Design review of the part built by this model. Coordinates are the model's own, in mm. Coordinates: 2 decimals unless noted, no trailing zeros. Loops run counter-clockwise (first coordinate to the right, second up) from the corner with the lowest first, then second, coordinate; pieces in that order, holes last. Notation, with made-up numbers: (86, -3) -> (103, -3) arc R4 ccw to (103, 3) -> close; hole circle Ø6 at (45, 85.5). An arc over 180 degrees is marked (long way). Answer in a Markdown table with one row per item.
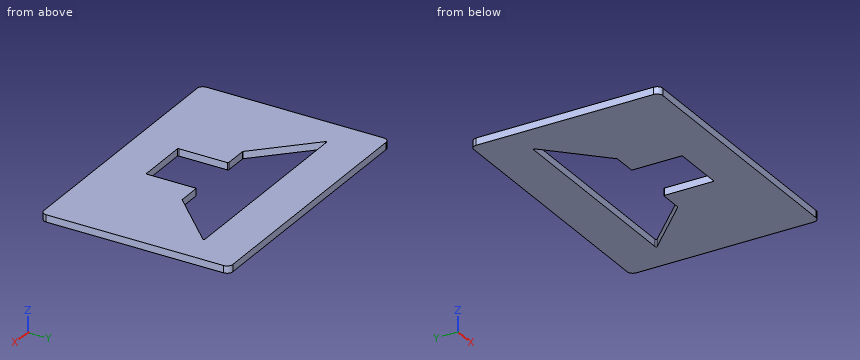
```python
from build123d import *

# Parameters (mm, degrees)
F1_DEPTH = 6.35
F3_DEPTH = 25.4
F5_DEPTH = 25.4


with BuildPart() as f1:
    # F0 (on Top) → F1 (new body)
    with BuildSketch(Plane.XY):
        with BuildLine():
            Line((113.9825, 84.1375), (-113.9825, 84.1375))
            ThreePointArc((-113.9825, 84.1375), (-117.574602, 82.649602), (-119.0625, 79.0575))
            Line((-119.0625, 79.0575), (-119.0625, -79.0575))
            ThreePointArc((-119.0625, -79.0575), (-117.574602, -82.649602), (-113.9825, -84.1375))
            Line((-113.9825, -84.1375), (113.9825, -84.1375))
            ThreePointArc((113.9825, -84.1375), (117.574602, -82.649602), (119.0625, -79.0575))
            Line((119.0625, -79.0575), (119.0625, 79.0575))
            ThreePointArc((119.0625, 79.0575), (117.574602, 82.649602), (113.9825, 84.1375))
        make_face()
    extrude(amount=F1_DEPTH)

    # F2 (on face) → F3 (cut)
    with BuildSketch(Plane.XY.offset(6.35)):
        Polygon((89.408, 43.8785), (0, 43.8785), (-89.408, 43.8785), (-44.45, -1.0795), (-22.479, -1.0795), (-22.479, -46.0375), (0, -46.0375), (22.479, -46.0375), (22.479, -1.0795), (44.45, -1.0795), align=None)
    extrude(amount=-F3_DEPTH, mode=Mode.SUBTRACT)

    # F4 (on face) → F5 (cut)
    with BuildSketch(Plane.XY.offset(6.35)):
        with BuildLine():
            ThreePointArc((-90.573099, 45.1485), (-91.300562, 44.662425), (-91.129875, 43.804324))
            Line((-91.129875, 43.804324), (-45.206675, -2.118876))
            ThreePointArc((-45.206675, -2.118876), (-44.951224, -2.289563), (-44.649899, -2.3495))
            Line((-44.649899, -2.3495), (-24.5364, -2.3495))
            ThreePointArc((-24.5364, -2.3495), (-23.979624, -2.580124), (-23.749, -3.1369))
            Line((-23.749, -3.1369), (-23.749, -46.5201))
            ThreePointArc((-23.749, -46.5201), (-23.518376, -47.076876), (-22.9616, -47.3075))
            Line((-22.9616, -47.3075), (22.9616, -47.3075))
            ThreePointArc((22.9616, -47.3075), (23.518376, -47.076876), (23.749, -46.5201))
            Line((23.749, -46.5201), (23.749, -3.1369))
            ThreePointArc((23.749, -3.1369), (23.979624, -2.580124), (24.5364, -2.3495))
            Line((24.5364, -2.3495), (44.649899, -2.3495))
            ThreePointArc((44.649899, -2.3495), (44.951224, -2.289563), (45.206675, -2.118876))
            Line((45.206675, -2.118876), (91.129875, 43.804324))
            ThreePointArc((91.129875, 43.804324), (91.300562, 44.662425), (90.573099, 45.1485))
            Line((90.573099, 45.1485), (-90.573099, 45.1485))
        make_face()
    extrude(amount=-F5_DEPTH, mode=Mode.SUBTRACT)


solid = f1.part
```
(1) To check wall thickness, follow probe 1 along Y at (x, z) = (-42, 3.5); probe 2 along Y at (x, z) = (19, 4.75); probe 3 along X at (y, z) = (20, 2.25). State the ranges of each line that lie inside material, in increasing order.
Evaluation:
| item | result |
|---|---|
| probe 1 | y = -84.14 to -2.35, 45.15 to 84.14 |
| probe 2 | y = -84.14 to -47.31, 45.15 to 84.14 |
| probe 3 | x = -119.06 to -67.33, 67.33 to 119.06 |
(2) Take a section at A-A on y = -32. Give the boundary of the cut face in (x, z), and give its area (3 significant figures).
Evaluation:
| item | result |
|---|---|
| outline | (-119.06, 0) -> (-23.75, 0) -> (-23.75, 6.35) -> (-119.06, 6.35) -> close; (23.75, 0) -> (119.06, 0) -> (119.06, 6.35) -> (23.75, 6.35) -> close |
| area | 1,210 mm² |
(3) Take a section at C-C on z = 2.5. Give the boundary of the cut face in (x, y), and give its area (3 significant figures).
Evaluation:
| item | result |
|---|---|
| outline | (-119.06, -79.06) arc R5.08 ccw to (-113.98, -84.14) -> (113.98, -84.14) arc R5.08 ccw to (119.06, -79.06) -> (119.06, 79.06) arc R5.08 ccw to (113.98, 84.14) -> (-113.98, 84.14) arc R5.08 ccw to (-119.06, 79.06) -> close; hole (-91.13, 43.8) -> (-45.21, -2.12) arc R0.79 ccw to (-44.65, -2.35) -> (-24.54, -2.35) arc R0.79 cw to (-23.75, -3.14) -> (-23.75, -46.52) arc R0.79 ccw to (-22.96, -47.31) -> (22.96, -47.31) arc R0.79 ccw to (23.75, -46.52) -> (23.75, -3.14) arc R0.79 cw to (24.54, -2.35) -> (44.65, -2.35) arc R0.79 ccw to (45.21, -2.12) -> (91.13, 43.8) arc R0.79 ccw to (90.57, 45.15) -> (-90.57, 45.15) arc R0.79 ccw to start |
| area | 31,400 mm² |
(4) Take a section at B-B on x = 8. Give the boundary of the cut face in (y, z).
Evaluation:
| item | result |
|---|---|
| outline | (-84.14, 0) -> (-47.31, 0) -> (-47.31, 6.35) -> (-84.14, 6.35) -> close; (45.15, 0) -> (84.14, 0) -> (84.14, 6.35) -> (45.15, 6.35) -> close |
